Autodesk Fusion 360 part; units mm, degrees
sketch "Sketch1" plane through (0, 0, 0) normal (0, 1, 0) x (1, 0, 0)
  line L0 (0, 0) -> (90, 0)
  line L1 (90, 0) -> (90, -26)
  line L2 (0, 0) -> (0, -26)
  line L3 (0, -26) -> (90, -26)
  dimension "d1" = 90
  dimension "d2" = 26
  dimension "d3" = 26
extrude "Extrude1" add sketch "Sketch1" along normal blind 5
sketch "Sketch2" plane through (0, 0, 0) normal (0, -1, 0) x (1, 0, 0)
  line L0 (0, 26) -> (0, 0)
  line L1 (0, 0) -> (90, 0)
  line L2 (90, 0) -> (90, 26)
  line L3 (90, 26) -> (0, 26)
  line L4 (0, 0) -> (90, 0)
  line L5 (90, 0) -> (90, 2)
  line L6 (0, 0) -> (0, 2)
  line L7 (0, 2) -> (90, 2)
  dimension "d6" = 2
  dimension "d7" = 2
extrude "Extrude2" add sketch "Sketch2" along normal blind 26 contours L0 L1 L2 L4 L5 L6 L7
sketch "Sketch3" plane through (0, 0, 0) normal (0, 0, -1) x (1, 0, 0)
  line L0 (0, 26) -> (0, -5)
  line L1 (0, -5) -> (90, -5)
  line L2 (90, -5) -> (90, 26)
  line L3 (90, 26) -> (0, 26)
  line L4 (90, 10.5) -> (0, 10.5) construction
  line L5 (45, 26) -> (45, -5) construction
  circle A0 centre (45, 10.5) radius 2.5
  dimension "d10" = 5
extrude "Extrude3" cut sketch "Sketch3" against normal blind 3 contours A0
sketch "Sketch4" plane through (0, 5, 0) normal (0, 1, 0) x (-1, 0, 0)
  line L0 (0, 0) -> (0, 26)
  line L1 (0, 26) -> (-90, 26)
  line L2 (-90, 26) -> (-90, 0)
  line L3 (-90, 0) -> (0, 0)
  line L4 (-90, 13) -> (0, 13) construction
  line L5 (-45, 26) -> (-45, 0) construction
  line L6 (-90, 7.6084) -> (-73, 7.6084) construction
  line L7 (-73, 7.6084) -> (-71.75, 7.6084) construction
  line L8 (-70.5, 7.6084) -> (-28.5, 7.6084) construction
  line L9 (-28.5, 7.6084) -> (-27.25, 7.6084) construction
  line L10 (-27.25, 7.6084) -> (-27.25, 13) construction
  line L11 (-71.75, 7.6084) -> (-71.75, 13) construction
  circle A0 centre (-27.25, 13) radius 1.25
  circle A1 centre (-71.75, 13) radius 1.25
  dimension "d13" = 17
  dimension "d15" = 1.25
  dimension "d17" = 42
  dimension "d18" = 1.25
  dimension "d20" = 2.5
  dimension "d21" = 2.5
sketch "Sketch5" plane through (0, 5, 0) normal (0, 1, 0) x (-1, 0, 0)
  line L0 (0, 0) -> (0, 26)
  line L1 (0, 26) -> (-90, 26)
  line L2 (-90, 26) -> (-90, 0)
  line L3 (-90, 0) -> (0, 0)
  line L4 (-90, 13) -> (0, 13) construction
  line L5 (-45, 0) -> (-45, 26) construction
  line L6 (-90, 19.9402) -> (0, 19.9402) construction
  line L7 (-35.0017, 26) -> (-35.0017, 0) construction
  line L8 (-54.9997, 26) -> (-54.9997, 0) construction
  circle A0 centre (-54.9997, 19.9402) radius 1.5
  circle A1 centre (-35.0017, 19.9402) radius 1.5
  line L9 (0, 6) -> (-90, 6) construction
  circle A2 centre (-35.0017, 6) radius 1.5
  circle A3 centre (-54.9997, 6) radius 1.5
  line L10 (-90, 13) -> (-62.75, 13) construction
  circle A4 centre (-62.75, 13) radius 1.25
  dimension "d24" = 3
  dimension "d25" = 3
  dimension "d27" = 3
  dimension "d28" = 3
  dimension "d29" = 27.25
  dimension "d30" = 2.5
extrude "Extrude5" cut sketch "Sketch5" against normal blind 5 contours A0 | A1 | A2 | A3 | A4
sketch "Sketch6" plane through (0, 5, 0) normal (0, 1, 0) x (-1, 0, 0)
  circle A0 centre (-54.9997, 19.9402) radius 1.5
  circle A1 centre (-54.9997, 6) radius 1.5
  circle A2 centre (-35.0017, 19.9402) radius 1.5
  circle A3 centre (-62.75, 13) radius 1.25
  circle A4 centre (-35.0017, 6) radius 1.5
  line L0 (0, 0) -> (0, 26)
  line L1 (0, 26) -> (-90, 26)
  line L2 (-90, 26) -> (-90, 0)
  line L3 (-90, 0) -> (0, 0)
  line L4 (0, 13) -> (-90, 13) construction
  line L5 (0, 9) -> (-27, 9) construction
  line L6 (-27, 9) -> (-27, 13) construction
  circle A5 centre (-27, 13) radius 1.25
  dimension "d33" = 27
  dimension "d34" = 2.5
extrude "Extrude6" cut sketch "Sketch6" against normal blind 5 contours A5
Model file for the job. Use its own axes, mm. A direction names the side the tool comes from. Round coordinates to 2 decimals unless told otherwise and drop trailing zeros. Write each loop counter-clockwise with the first axis right and the second up, starting at its lowest first coordinate (ties: lowest second). Pieces come first, ordered by that corner, then holes. Notation, with made-up numbers: (-33.75, 23) - (9.25, 23) arc R30 ccw to (9.25, 47) - close; hole circle Ø4 at (30.5, -37). An arc over 180 degrees is marked (long way). One line per item, written item: value.
(1) Cut at D-D, the plane x = 45. Give the cut face in (y, z), plus the area to 3 significant figures.
Values follow:
outline: (-26, 0) - (-13, 0) - (-13, 2) - (-26, 2) - close; (-8, 0) - (5, 0) - (5, 26) - (0, 26) - (0, 2) - (-8, 2) - close
area: 172 mm²
(2) Drop flat-ended pins along their axis: P1, Ø4, axis at x = 56.5, y = -6, coming from the +Z side; P2, Ø5, axis at x = 35, z = 6, coming from the -Y side. Give the stop position or say it passes through.
Values follow:
P1: stops at z = 2
P2: stops at y = 0
(3) Cut at A-A, the plane y = -10.5. Give the cut face in (x, z).
Values follow:
outline: (0, 0) - (42.5, 0) - (42.5, 2) - (0, 2) - close; (47.5, 0) - (90, 0) - (90, 2) - (47.5, 2) - close
(4) Cut at B-B, the plane x = 62.75. Give the cut face in (y, z), plus the area to 4 significant figures.
Values follow:
outline: (-26, 0) - (5, 0) - (5, 11.75) - (0, 11.75) - (0, 2) - (-26, 2) - close; (0, 14.25) - (5, 14.25) - (5, 26) - (0, 26) - close
area: 169.5 mm²
(5) Cut at C-C, the plane z = 6. Give the cut face in (x, y).
Values follow:
outline: (0, 0) - (33.5, 0) - (33.5, 5) - (0, 5) - close; (36.5, 0) - (53.5, 0) - (53.5, 5) - (36.5, 5) - close; (56.5, 0) - (90, 0) - (90, 5) - (56.5, 5) - close
(6) 3-axis set-ups, long thin cutter, end or side, ignore diameter. For faces 1 (the cylindrical face through (61.56, 2.54, 13.38)), 2 (the flat face through (44, -16, 2)): which of +Z, -Z, +X, -X, +Y, -Y reach the whole face in a straight line?
Values follow:
face 1: +Y, -Y
face 2: +Z, +X, -X, -Y
(7) Wall check: probe 1 along X at (y, z) = (3.5, 20.5); probe 2 along X at (y, z) = (-10.5, 0.8); probe 3 along Y at (x, z) = (45, 1). Give the ranges that are in metal, low to high.
Values follow:
probe 1: x = 0 to 33.61, 36.39 to 53.61, 56.39 to 90
probe 2: x = 0 to 42.5, 47.5 to 90
probe 3: y = -26 to -13, -8 to 5
(8) Two-plate mould, pull along X, no slides. Class faces 3 (the flat face through (90, 1, 9)), 4 (the flat face through (44, 2, 26)), 5 (the flat face through (0, 1, 9)), 6 (the cylindrical face through (53.57, 2.54, 20.39)): pulls with the +X half, pulls with the -X half, needs draft (parallel to the pull), parting line crosses it, or undercut.
Values follow:
face 3: pulls with the +X half
face 4: needs draft
face 5: pulls with the -X half
face 6: undercut
